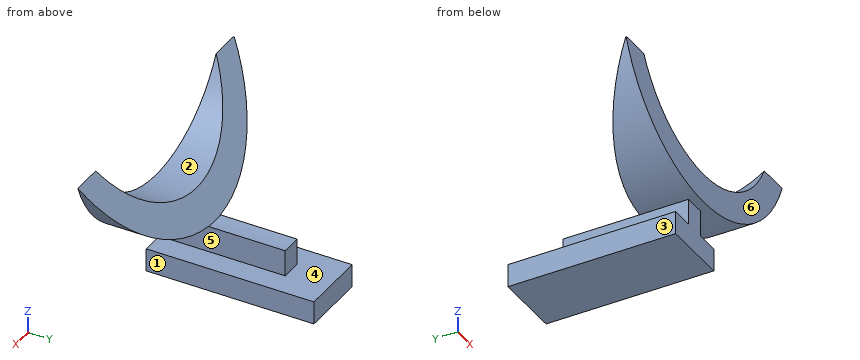
```python
from build123d import *

# Parameters (mm, degrees)
SKETCH1_W               = 16
SKETCH1_H               = 5
BOSS_EXTRUDE1_DEPTH     = 30
BOSS_EXTRUDE2_START     = -2.25
BOSS_EXTRUDE2_DEPTH     = 14
CUT_EXTRUDE1_DEPTH      = 33.691742077
CUT_EXTRUDE1_DEPTH_BACK = 33.691742077
BOSS_EXTRUDE3_START     = 30
SKETCH1_3_W             = 16
SKETCH1_3_H             = 5
BOSS_EXTRUDE3_DEPTH     = 10
SKETCH5_W               = 16
SKETCH5_H               = 0.5
BOSS_EXTRUDE4_DEPTH     = 40


with BuildPart() as part:
    # Sketch1 → Boss-Extrude1 (new body)
    with BuildSketch(Plane(origin=(0, 0, 0), x_dir=(1, 0, 0), z_dir=(0, 1, 0))):
        Rectangle(SKETCH1_W, SKETCH1_H)
        with BuildLine():
            Line((2.5, -9.25), (2.5, -2.5))
            Line((2.5, -2.5), (-2.5, -2.5))
            Line((-2.5, -2.5), (-2.5, -9.25))
            ThreePointArc((-2.5, -9.25), (0, -9.160600109), (2.5, -9.25))
        make_face()
    extrude(amount=BOSS_EXTRUDE1_DEPTH)

    # Sketch2 → Boss-Extrude2 (add)
    with BuildSketch(Plane(origin=(0, 0, 0), x_dir=(1, 0, 0), z_dir=(0, 1, 0)).offset(BOSS_EXTRUDE2_START)):
        with BuildLine():
            ThreePointArc((32.691742077, -31.660600109), (0, -9.160600109), (-32.691742077, -31.660600109))
            Line((-32.691742077, -31.660600109), (-25.194555463, -31.660600109))
            ThreePointArc((-25.194555463, -31.660600109), (0, -16.035600109), (25.194555463, -31.660600109))
            Line((25.194555463, -31.660600109), (32.691742077, -31.660600109))
        make_face()
    extrude(amount=BOSS_EXTRUDE2_DEPTH)

    # Sketch3 → Cut-Extrude1 (cut, two sides)
    with BuildSketch(Plane(origin=(0, 0, 0), x_dir=(0, 0, -1), z_dir=(1, 0, 0))) as cut_extrude1_sk:
        Polygon((-31.660600109, -2.25), (-31.660600109, 11.75), (-9.160600109, 11.75), align=None)
    extrude(amount=CUT_EXTRUDE1_DEPTH, mode=Mode.SUBTRACT)
    extrude(cut_extrude1_sk.sketch, amount=-CUT_EXTRUDE1_DEPTH_BACK, mode=Mode.SUBTRACT)

    # Sketch1_3 → Boss-Extrude3 (add)
    with BuildSketch(Plane(origin=(0, 0, 0), x_dir=(1, 0, 0), z_dir=(0, 1, 0)).offset(BOSS_EXTRUDE3_START)):
        Rectangle(SKETCH1_3_W, SKETCH1_3_H)
    extrude(amount=BOSS_EXTRUDE3_DEPTH)

    # Sketch5 → Boss-Extrude4 (add)
    with BuildSketch(Plane(origin=(0, 40, 0), x_dir=(1, 0, 0), z_dir=(0, 1, 0))):
        with Locations((0, -2.75)):
            Rectangle(SKETCH5_W, SKETCH5_H)
    extrude(amount=-BOSS_EXTRUDE4_DEPTH)


solid = part.part
```
Verification items for the finished model (mm, model axes). Face numbers are marked on the shaded views. A direction names the side the tool comes from. Coordinates: 2 decimals unless noted, no trailing zeros. Loops run counter-clockwise (first coordinate to the right, second up) from the corner with the lowest first, then second, coordinate; pieces in that order, holes last. Notation, with made-up numbers: (-36, -16) -> (8, -16) arc R24 ccw to (8, -5) -> close; hole circle Ø4 at (67, -11). An arc over 180 degrees is marked (long way). Put each result on its own line as item: value.
1. Thickness scan on line 1 (Z direction, x = -3, y = 4); line 2 (X direction, y = 24, z = 2.5); line 3 (Z direction, x = -1, y = 12). Record the ranges inside material, lowest first.
Result set:
line 1: z = -2.5 to 3, 9.29 to 16.2
line 2: x = -8 to 8
line 3: z = -2.5 to 9.17
2. Section check C-C, the plane z = 23.5. Record the boundary of the cut face in (x, y).
Result set:
outline: (-28.25, -2.25) -> (-19.08, -2.25) -> (-19.08, 2.83) -> (-28.25, 2.83) -> close; (19.08, -2.25) -> (28.25, -2.25) -> (28.25, 2.83) -> (19.08, 2.83) -> close
3. Gauge pin test, flat ends, axial feed: P1, Ø3, axis at y = 11, z = 0.5, coming from the -X side; P2, Ø1.9, axis at y = 11.5, z = 7, coming from the +X side; P3, Ø1.5, axis at y = 13, z = 4, coming from the -X side. Record the tip position at first contact, or that the pin passes through.
Result set:
P1: stops at x = -8
P2: stops at x = 2.5
P3: stops at x = -2.5
4. Mould release check, pull along X, two halves, no side actions. Record for the marked faces 1, 2, 3 and 4: pulls with the +X half, pulls with the -X half, needs draft (parallel to the pull), parting line crosses it, or undercut.
Result set:
face 1: pulls with the +X half
face 2: undercut
face 3: pulls with the -X half
face 4: needs draft
5. Section check B-B, the plane z = 19.5. Record the boundary of the cut face in (x, y).
Result set:
outline: (-24.84, -2.25) -> (-13.52, -2.25) -> (-13.52, 5.32) -> (-24.84, 5.32) -> close; (13.52, -2.25) -> (24.84, -2.25) -> (24.84, 5.32) -> (13.52, 5.32) -> close
6. Tool access check on the marked faces 5 and 6. Record the directions out of +Z, -Z, +X, -X, +Y, -Y that give a thin tool (end or side, any length) a straight path to the whole face; none if there is none.
Result set:
face 5: +X, +Y, -Y
face 6: +Z, -Z, +X, -X, -Y
7. Section check A-A, the plane y = 19. Record the boundary of the cut face in (x, z), then the cut area to 3 significant figures.
Result set:
outline: (-8, -2.5) -> (8, -2.5) -> (8, 3) -> (2.5, 3) -> (2.5, 9.25) arc R35 cw to (-2.5, 9.25) -> (-2.5, 3) -> (-8, 3) -> close
area: 119 mm^2
8. Section check D-D, the plane z = 2. Record the boundary of the cut face in (x, y).
Result set:
outline: (-8, 0) -> (8, 0) -> (8, 40) -> (-8, 40) -> close
